Study the drawing (mm; zero at the part's minimum x, y, z) and answer. A direction names the side the tool comes from. Coordinates: 2 decimals unless noted, no trailing zeros. Write each loop counter-clockwise with the first axis right and the second up, starting at its lowest first coordinate (ties: lowest second). Pieces come first, ordered by that corner, then holes. Notation, with made-up numbers: (-11, 60.5) -> (17, 60.5) arc R23 cw to (17, 86.5) -> close; hole circle Ø10 at (16.5, -25). An arc over 180 degrees is marked (long way). Answer in a Markdown table with one row per item. Add a question column.
Item 1: Section B-B on z = 60 is taken. Write down the section's boundary in (x, y).
Item 2: Section C-C on x = 60 is taken. Write down the section's boundary in (y, z), then the cut area to 3 significant figures.
Item 3: Straight lines are drawn through the part: line 1 (X direction, y = 40, z = 60); line 2 (X direction, y = 5.5, z = 36.5); line 3 (Z direction, x = 54.5, y = 10). For each, find the intervals that lie inside material, in ascending order. Write a range as from..to.
Item 4: Section A-A on y = 28.5 is taken. Write down the section's boundary in (x, z).
Item 5: Given pin 1 Ø23 at (x, z) = (60, 60) entering from -Y; pin 2 Ø2 at (x, y) = (63.5, 20.5) entering from -Z; pin 3 Ø21.5 at (x, y) = (30, 32) entering from -Z, each flat-ended and moving along its own axis, determine where each tip first touches the part or whether it passes through.
Item 6: Section D-D on z = 45 is taken. Write down the section's boundary in (x, y), then the cut area to 3 significant figures.
Item 7: For a pull along Y with two mould halves and no side action, classify the marked faces 4, 5, 6 and 7 as +Y half, -Y half, draft (parallel to the pull), parting line (faces both ways), or undercut.
Item 8: Which of the six approach directions +Z, -Z, +X, -X, +Y, -Y give full straight-line access (tool end or side, diameter ignored) to the marked faces 1, 2 and 3?
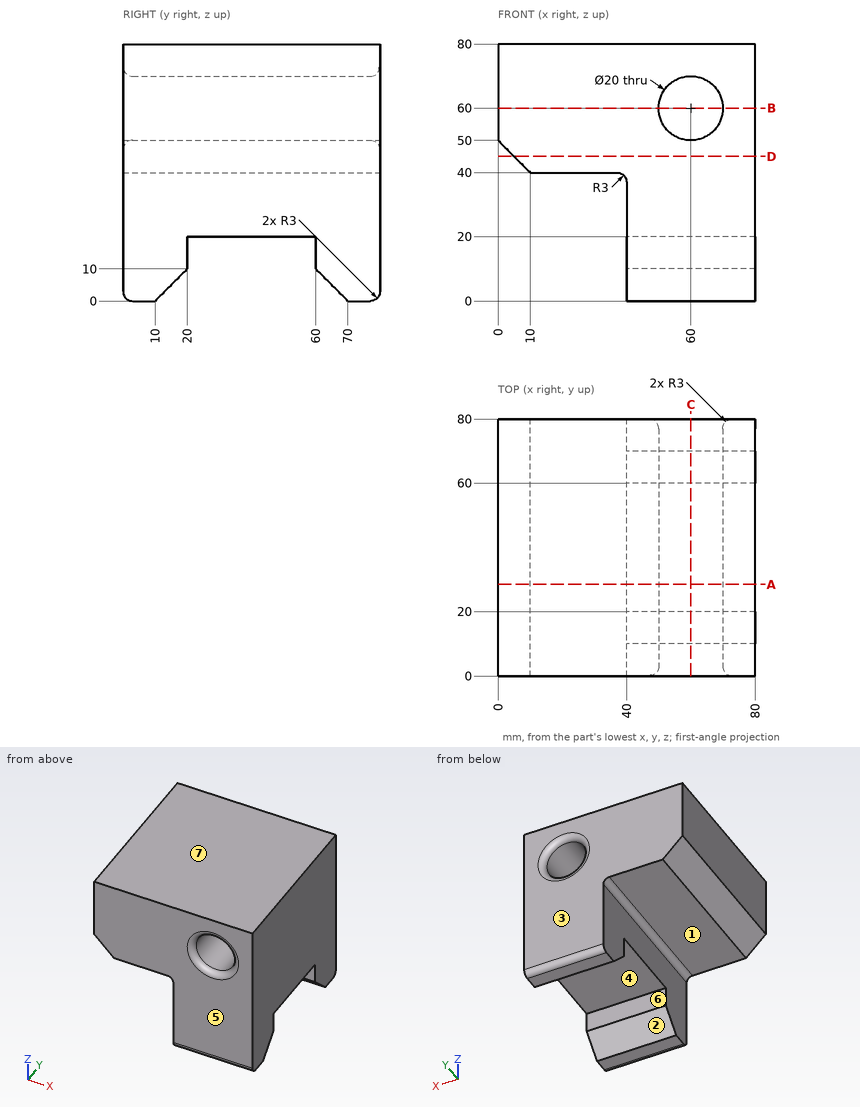
Results below:
| question | item | result |
|---|---|---|
| 1 | outline | (0, 0) -> (47, 0) arc R3 ccw to (50, 3) -> (50, 77) arc R3 ccw to (47, 80) -> (0, 80) -> close; (70, 3) arc R3 ccw to (73, 0) -> (80, 0) -> (80, 80) -> (73, 80) arc R3 ccw to (70, 77) -> close |
| 2 | outline | (0, 3) arc R3 ccw to (3, 0) -> (10, 0) -> (20, 10) -> (20, 20) -> (60, 20) -> (60, 10) -> (70, 0) -> (77, 0) arc R3 ccw to (80, 3) -> (80, 47) arc R3 ccw to (77, 50) -> (3, 50) arc R3 ccw to (0, 47) -> close; (0, 73) arc R3 ccw to (3, 70) -> (77, 70) arc R3 ccw to (80, 73) -> (80, 80) -> (0, 80) -> close |
| 2 | area | 3,890 mm2 |
| 3 | line 1 | x = 0..50, 70..80 |
| 3 | line 2 | x = 40..80 |
| 3 | line 3 | z = 0..51.65, 68.35..80 |
| 4 | outline | (0, 50) -> (10, 40) -> (37, 40) arc R3 cw to (40, 37) -> (40, 20) -> (80, 20) -> (80, 80) -> (0, 80) -> close; hole circle Ø20 at (60, 60) |
| 5 | pin 1 | stops at y = 0.4 |
| 5 | pin 2 | stops at z = 9.5 |
| 5 | pin 3 | stops at z = 20 |
| 6 | outline | (5, 0) -> (80, 0) -> (80, 80) -> (5, 80) -> close |
| 6 | area | 6,000 mm2 |
| 7 | face 4 | undercut |
| 7 | face 5 | -Y half |
| 7 | face 6 | undercut |
| 7 | face 7 | draft |
| 8 | face 1 | -Z, -X, +Y, -Y |
| 8 | face 2 | -Z, +X, -X |
| 8 | face 3 | +Z, -Z, +X, -X, +Y |
